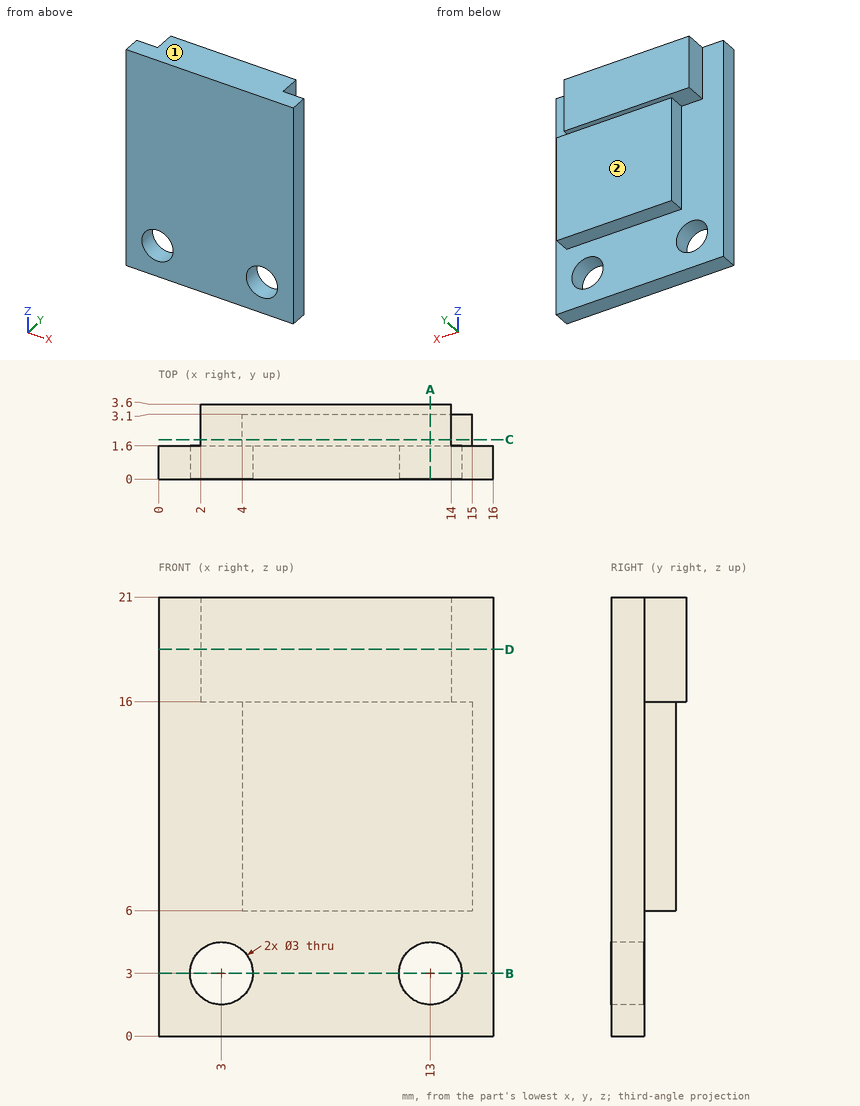
Design review of the part shown in the three views and the two pictorial views. Dimensions are in mm from the part's minimum x, y and z. A direction names the side the tool comes from. Round coordinates to 2 decimals unless told otherwise and drop trailing zeros. Order: outer loops, then holes, each group sorted by start corner. A loop starts at its lowest first (then second) coordinate and runs counter-clockwise, first axis right, second up.
Item 1: Add section B-B, the plane z = 3. State the section outline as (x, y) points, and give its area (3 significant figures).
Working result:
outline: (0, 0) - (1.5, 0) - (1.5, 1.6) - (0, 1.6) - close; (4.5, 0) - (11.5, 0) - (11.5, 1.6) - (4.5, 1.6) - close; (14.5, 0) - (16, 0) - (16, 1.6) - (14.5, 1.6) - close
area: 16.0 mm2
Item 2: Add section A-A, the plane x = 13. State the section outline as (y, z) points.
Working result:
outline: (0, 0) - (1.6, 0) - (1.6, 1.5) - (0, 1.5) - close; (0, 4.5) - (1.6, 4.5) - (1.6, 6) - (3.1, 6) - (3.1, 16) - (3.6, 16) - (3.6, 21) - (0, 21) - close
Item 3: To check wall thickness, follow probe 1 along X at (y, z) = (0.35, 3); probe 2 along Y at (x, z) = (1, 12.25); probe 3 along X at (y, z) = (2.2, 8). State the ranges of each line that lie inside material, in increasing order.
Working result:
probe 1: x = 0 to 1.5, 4.5 to 11.5, 14.5 to 16
probe 2: y = 0 to 1.6
probe 3: x = 4 to 15
Item 4: Machinability: for the marked faces 1 and 2, which of the approach directions +Z, -Z, +X, -X, +Y, -Y give a long, thin tool a straight path to every point of the face, cutting with its end or side? Answer none if there is none.
Working result:
face 1: +Z, +X, -X, +Y, -Y
face 2: -Z, +X, -X, +Y
Item 5: Add section C-C, the plane y = 1.9. State the section outline as (x, z) points.
Working result:
outline: (2, 16) - (4, 16) - (4, 6) - (15, 6) - (15, 16) - (14, 16) - (14, 21) - (2, 21) - close
Item 6: For pin 1 (1.6 mm diameter, centred on y = 2.5, z = 10.5, fed in from +X); pin 2 (1.6 mm diameter, centred on x = 5.5, y = 2.5, fed in from -Z); pin 3 (4 mm diameter, centred on x = 9, z = 6, fed in from +Y); pin 4 (2.5 mm diameter, centred on x = 3, z = 3, fed in from +Y), all flat-tipped, find the tip position at first contact; note any pin that passes through.
Working result:
pin 1: stops at x = 15
pin 2: stops at z = 6
pin 3: stops at y = 3.1
pin 4: passes through
Item 7: Add section D-D, the plane z = 18.5. State the section outline as (x, y) points.
Working result:
outline: (0, 0) - (16, 0) - (16, 1.6) - (14, 1.6) - (14, 3.6) - (2, 3.6) - (2, 1.6) - (0, 1.6) - close
